Model file for the job. Use its own axes, mm. A direction names the side the tool comes from. Give positions to 0.01 mm unless a question says otherwise; leave off trailing zeros. Loops run counter-clockwise (first coordinate to the right, second up) from the corner with the lowest first, then second, coordinate; pieces in that order, holes last. Notation, with made-up numbers: (5, 30) - (57, 30) arc R22 cw to (57, 42) - close; hole circle Ø7 at (51.5, 56.25). An arc over 180 degrees is marked (long way). Answer as CSV lines item,"result". Start each with the question number.
Item 1: Drill centre lines: L1, parallel to X at y = -2.75, z = -3.35; L2, parallel to Y at x = 76, z = -3.9. Where is each one in solid material? Low to high. Write a range as from..to.
Item 2: Saw through at B-B on z = -2.1. Give the cut face in (x, y).
Item 3: Saw through at A-A on y = -4.5. Give the cut face in (x, z).
Item 4: Pin check, flat tips, straight feed: pin 1 (1.8 mm diameter, centred on y = -4, z = -1.5, fed in from -X); pin 2 (1.8 mm diameter, centred on x = 34.5, z = -2, fed in from -Y). Stop position of each tip, or through.
Item 5: Tool access for faces 5 (the flat face through (130, 3, -3)), 6 (the flat face through (-117, -1, -3)), 7 (the flat face through (-97, -7, -3)), 8 (the flat face through (117, -1, -3)), 9 (the flat face through (52.286, -4, -3)): list every direction of +Z, -Z, +X, -X, +Y, -Y with a clear straight run to the whole face (end or side of a thin tool).
Item 6: Saw through at C-C on x = -109.5. Give the cut face in (y, z).
Item 7: Pull direction X, two halves, no side cores. Call faces 1 (the flat face through (-2, 2, 0)), 2 (the flat face through (-13.429, -4, -3)), 3 (the flat face through (-103.143, -4, -3)), 4 (the flat face through (-52.286, -4, -3)): pulls with the +X half, pulls with the -X half, needs draft (parallel to the pull), parting line crosses it, or undercut.
from build123d import *

# Parameters (mm, degrees)
SKETCH1_W           = 260
SKETCH1_H           = 14
BOSS_EXTRUDE1_DEPTH = 6
SKETCH3_W           = 26.857142857
SKETCH3_H           = 6
SKETCH3_W_2         = 13.428571429
CUT_EXTRUDE1_DEPTH  = 7


with BuildPart() as part:
    # Sketch1 → Boss-Extrude1 (new body)
    with BuildSketch(Plane.XY):
        Rectangle(SKETCH1_W, SKETCH1_H)
    extrude(amount=-BOSS_EXTRUDE1_DEPTH)

    # Sketch3 → Cut-Extrude1 (cut, through all)
    with BuildSketch(Plane.XY):
        with Locations((-116.571428572, -4)):
            Rectangle(SKETCH3_W, SKETCH3_H)
        with Locations((-77.714285714, -4)):
            Rectangle(SKETCH3_W, SKETCH3_H)
        with Locations((-38.857142858, -4)):
            Rectangle(SKETCH3_W, SKETCH3_H)
        with Locations((-6.714285715, -4)):
            Rectangle(SKETCH3_W_2, SKETCH3_H)
    cut_extrude1 = extrude(amount=-CUT_EXTRUDE1_DEPTH, mode=Mode.SUBTRACT)

    # Mirror1: Cut-Extrude1 across plane
    add(cut_extrude1.mirror(Plane(origin=(0, 0, 0), x_dir=(0, 0, 1), z_dir=(1, 0, 0))), mode=Mode.SUBTRACT)


solid = part.part
Responses:
1,L1,"-103.14..-91.14, -64.29..-52.29, -25.43..-13.43, 13.43..25.43, 52.29..64.29, 91.14..103.14"
1,L2,"-1..7"
2,outline,"(-130, -1) - (-103.14, -1) - (-103.14, -7) - (-91.14, -7) - (-91.14, -1) - (-64.29, -1) - (-64.29, -7) - (-52.29, -7) - (-52.29, -1) - (-25.43, -1) - (-25.43, -7) - (-13.43, -7) - (-13.43, -1) - (13.43, -1) - (13.43, -7) - (25.43, -7) - (25.43, -1) - (52.29, -1) - (52.29, -7) - (64.29, -7) - (64.29, -1) - (91.14, -1) - (91.14, -7) - (103.14, -7) - (103.14, -1) - (130, -1) - (130, 7) - (-130, 7) - close"
3,outline,"(-103.14, -6) - (-91.14, -6) - (-91.14, 0) - (-103.14, 0) - close; (-64.29, -6) - (-52.29, -6) - (-52.29, 0) - (-64.29, 0) - close; (-25.43, -6) - (-13.43, -6) - (-13.43, 0) - (-25.43, 0) - close; (13.43, -6) - (25.43, -6) - (25.43, 0) - (13.43, 0) - close; (52.29, -6) - (64.29, -6) - (64.29, 0) - (52.29, 0) - close; (91.14, -6) - (103.14, -6) - (103.14, 0) - (91.14, 0) - close"
4,pin 1,"x = -103.14"
4,pin 2,"y = -1"
5,face 5,"+Z, -Z, +X, +Y, -Y"
5,face 6,"+Z, -Z, -X, -Y"
5,face 7,"+Z, -Z, +X, -X, -Y"
5,face 8,"+Z, -Z, +X, -Y"
5,face 9,"+Z, -Z, -Y"
6,outline,"(-1, -6) - (7, -6) - (7, 0) - (-1, 0) - close"
7,face 1,"needs draft"
7,face 2,"undercut"
7,face 3,"pulls with the -X half"
7,face 4,"undercut"
